Autodesk Inventor part; units mm, degrees
ref_plane "YZ Plane" through (0, 0, 0) normal (1, 0, 0) x (0, 1, 0)
ref_plane "XZ Plane" through (0, 0, 0) normal (0, 1, 0) x (-1, 0, 0)
ref_plane "XY Plane" through (0, 0, 0) normal (0, 0, 1) x (1, 0, 0)
sketch "Sketch1" plane through (0, 0, 0) normal (1, 0, 0) x (0, 1, 0)
  line L0 (-14.1111, 2.4111) -> (-14.1111, -16.5889)
  line L1 (7.8889, -16.5889) -> (7.8889, 2.4111)
  arc A0 (7.8889, 2.4111) -> (-0.1111, 2.4111) centre (3.8889, 2.4111) ccw
  arc A1 (-0.1111, -16.5889) -> (7.8889, -16.5889) centre (3.8889, -16.5889) ccw
  line L2 (-0.1111, 2.4111) -> (-14.1111, 2.4111)
  line L3 (-0.1111, -16.5889) -> (-14.1111, -16.5889)
  line L4 (7.3889, -10.0889) -> (0.3889, -10.0889)
  line L5 (7.3889, -13.0889) -> (0.3889, -13.0889)
  line L6 (7.3889, -4.0889) -> (0.3889, -4.0889)
  line L7 (7.3889, -1.0889) -> (0.3889, -1.0889)
  line L8 (7.3889, 2.4111) -> (7.3889, -16.5889)
  arc A2 (0.3889, -16.5889) -> (7.3889, -16.5889) centre (3.8889, -16.5889) ccw
  arc A3 (7.3889, 2.4111) -> (0.3889, 2.4111) centre (3.8889, 2.4111) ccw
  line L9 (0.3889, 2.4111) -> (0.3889, -16.5889)
  circle A4 centre (3.8889, 2.4111) radius 2
  circle A5 centre (3.8889, -16.5889) radius 2
  point P0 (0, 0)
  dimension "d5" = 0.5
  dimension "d6" = 4
  dimension "d7" = 4
extrude "Extrusion1" add sketch "Sketch1" along normal blind 1.5 contours L2 A0 L1 A1 L3 L0 | L8 L5 L9 L4 | L4 L9 L6 L8 | L6 L9 L7 L8 | L8 A2 L9 L5 | L7 L9 A3 L8
extrude "Extrusion2" add sketch "Sketch1" along normal blind 3 contours L8 L5 L9 L4 | L4 L9 L6 L8 | L6 L9 L7 L8 | L8 A2 L9 L5 | L7 L9 A3 L8
extrude "Extrusion3" add sketch "Sketch1" along normal blind 12 contours L8 L5 L9 L4 | L6 L9 L7 L8
properties part number "HC020K"
Part model, mm, in its own coordinate system. A direction names the side the tool comes from. Round coordinates to 2 decimals unless told otherwise and drop trailing zeros. Loops run counter-clockwise (first coordinate to the right, second up) from the corner with the lowest first, then second, coordinate; pieces in that order, holes last. Notation, with made-up numbers: (-30, 79) -> (0, 79) arc R20 ccw to (0, 92) -> close; hole circle Ø4 at (69, 26.25). An arc over 180 degrees is marked (long way). Use one line per item in the form item = value. Start each with the question number.
Item 1: Band-saw the part on C-C (z = -10.5). List the corners of the cut face in (x, y), plus the area to 4 significant figures.
Item 2: Band-saw the part on A-A (y = 3). List the corners of the cut face in (x, z).
Item 3: Drop flat-ended pins along their axis: pin 1 Ø4 at (x, z) = (9.5, -8) entering from +Y; pin 2 Ø3 at (x, z) = (9.5, -10.5) entering from +Y; pin 3 Ø1.2 at (x, y) = (1, -8.5) entering from -Z; pin 4 Ø2 at (x, y) = (5.5, 2) entering from -Z. Give the stop position or say it passes through.
Item 4: Band-saw the part on B-B (x = 6.5). List the corners of the cut face in (y, z).
Item 5: Drill centre lines: line 1 along Z through (x, y) = (7, 2.75); line 2 along Z through (x, y) = (2.75, 2.75); line 3 along Z through (x, y) = (0.75, -6). Where is each one in solid material? Low to high.
Item 6: Tool access for faces 5 (the flat face through (1, -7, -16.589)), 6 (the flat face through (7, 4, -1.089)), 7 (the cylindrical face through (2.24, 3.966, -20.088)): list every direction of +Z, -Z, +X, -X, +Y, -Y with a clear straight run to the whole face (end or side of a thin tool).
Item 7: Two-plate mould, pull along Z, no slides. Class faces 1 (the cylindrical face through (0.74, 3.8, 6.41)), 2 (the flat face through (3, 4, -7)), 3 (the flat face through (7, 4, -4.089)), 4 (the flat face through (12, 4, -12)): released by +Z, released by -Z, zero draft, split by the parting line, or undercut.
Item 8: Band-saw the part on D-D (z = -17.25). List the corners of the cut face in (x, y).
Data:
q1.outline = (0, -14.11) -> (1.5, -14.11) -> (1.5, 0.39) -> (12, 0.39) -> (12, 7.39) -> (1.5, 7.39) -> (1.5, 7.89) -> (0, 7.89) -> close
q1.area = 106.5 mm^2
q2.outline = (0, -20.49) -> (1.5, -20.49) -> (1.5, -19.97) -> (3, -19.97) -> (3, -18.38) -> (0, -18.38) -> close; (0, -14.8) -> (3, -14.8) -> (3, -13.09) -> (12, -13.09) -> (12, -10.09) -> (3, -10.09) -> (3, -4.09) -> (12, -4.09) -> (12, -1.09) -> (3, -1.09) -> (3, 0.62) -> (0, 0.62) -> close; (0, 4.2) -> (3, 4.2) -> (3, 5.8) -> (1.5, 5.8) -> (1.5, 6.31) -> (0, 6.31) -> close
q3.pin_1 = through
q3.pin_2 = 7.39
q3.pin_3 = -16.59
q3.pin_4 = -13.09
q4.outline = (0.39, -13.09) -> (7.39, -13.09) -> (7.39, -10.09) -> (0.39, -10.09) -> close; (0.39, -4.09) -> (7.39, -4.09) -> (7.39, -1.09) -> (0.39, -1.09) -> close
q5.line_1 = -13.09 to -10.09, -4.09 to -1.09
q5.line_2 = -19.9 to -18.23, -14.94 to 0.77, 4.06 to 5.72
q5.line_3 = -16.59 to 2.41
q6.face_5 = -Z, +X, -X, -Y
q6.face_6 = +Z, +X, +Y, -Y
q6.face_7 = -Z, +X
q7.face_1 = released by +Z
q7.face_2 = undercut
q7.face_3 = undercut
q7.face_4 = zero draft
q8.outline = (0, -0.06) -> (1.5, -0.06) -> (1.5, 0.45) -> (3, 0.45) -> (3, 2) -> (0, 2) -> close; (0, 5.78) -> (3, 5.78) -> (3, 7.33) -> (1.5, 7.33) -> (1.5, 7.83) -> (0, 7.83) -> close
